Source: CAD feature listing. Evaluate the final solid. Frame: model axes, mm. Give positions to 0.01 mm unless a question says otherwise; leave off trailing zeros. Order: outer loops, then holes, each group sorted by start corner. A loop starts at its lowest first (then second) coordinate and runs counter-clockwise, first axis right, second up.
from build123d import *

# Parameters (mm, degrees)
BOSS_EXTRUDE1_DEPTH = 3.81
SKETCH2_R           = 3.175
CUT_EXTRUDE1_DEPTH  = 85.852


with BuildPart() as part:
    # Sketch1 → Boss-Extrude1 (new body)
    with BuildSketch(Plane(origin=(0, 0, 0), x_dir=(1, 0, 0), z_dir=(0, 1, 0))):
        with BuildLine():
            Line((-106.328404832, 71.61361972), (-235.457093287, 71.61361972))
            ThreePointArc((-235.457093287, 71.61361972), (-253.237093287, 53.83361972), (-235.457093287, 36.05361972))
            Line((-235.457093287, 36.05361972), (-215.137093287, 36.05361972))
            ThreePointArc((-215.137093287, 36.05361972), (-211.544990839, 34.565722168), (-210.057093287, 30.97361972))
            Line((-210.057093287, 30.97361972), (-210.057093287, -116.34638028))
            ThreePointArc((-210.057093287, -116.34638028), (-211.544990839, -119.938482729), (-215.137093287, -121.42638028))
            Line((-215.137093287, -121.42638028), (-235.457093287, -121.42638028))
            ThreePointArc((-235.457093287, -121.42638028), (-253.237093287, -139.20638028), (-235.457093287, -156.98638028))
            Line((-235.457093287, -156.98638028), (-106.328404832, -156.98638028))
            Line((-106.328404832, -156.98638028), (160.782906713, -156.98638028))
            Line((160.782906713, -156.98638028), (186.182906713, -156.98638028))
            ThreePointArc((186.182906713, -156.98638028), (203.962906713, -139.20638028), (186.182906713, -121.42638028))
            Line((186.182906713, -121.42638028), (165.862906713, -121.42638028))
            ThreePointArc((165.862906713, -121.42638028), (162.270804264, -119.938482729), (160.782906713, -116.34638028))
            Line((160.782906713, -116.34638028), (160.782906713, 30.97361972))
            ThreePointArc((160.782906713, 30.97361972), (162.270804264, 34.565722168), (165.862906713, 36.05361972))
            Line((165.862906713, 36.05361972), (186.182906713, 36.05361972))
            ThreePointArc((186.182906713, 36.05361972), (203.962906713, 53.83361972), (186.182906713, 71.61361972))
            Line((186.182906713, 71.61361972), (160.782906713, 71.61361972))
            Line((160.782906713, 71.61361972), (-106.328404832, 71.61361972))
        make_face()
    extrude(amount=BOSS_EXTRUDE1_DEPTH)

    # Sketch2 → Cut-Extrude1 (cut)
    with BuildSketch(Plane(origin=(0, 3.81, 0), x_dir=(1, 0, 0), z_dir=(0, 1, 0))):
        with Locations((-235.457093287, 53.83361972)):
            Circle(SKETCH2_R)
        with Locations((186.182906713, 53.83361972)):
            Circle(SKETCH2_R)
        with Locations((186.182906713, -139.20638028)):
            Circle(SKETCH2_R)
        with Locations((-235.457093287, -139.20638028)):
            Circle(SKETCH2_R)
    extrude(amount=-CUT_EXTRUDE1_DEPTH, mode=Mode.SUBTRACT)


solid = part.part
1) First-contact query: pin 1 Ø4 at (x, z) = (-235.46, 139.21) entering from +Y; pin 2 Ø5 at (x, z) = (-48, -15.5) entering from -Y. Flat tips, straight axial feed; report the tip coordinate or a pass-through.
Checks:
pin 1: passes through
pin 2: stops at y = 0
2) Section query C-C on z = 127. Output: boundary loops of the cut face in (x, y), and give its area (3 significant figures).
Checks:
outline: (-248.39, 0) - (199.11, 0) - (199.11, 3.81) - (-248.39, 3.81) - close
area: 1,700 mm2
3) Ray query, L1, parallel to X at y = 0.9, z = 142; L2, parallel to X at y = 2, z = -16; L3, parallel to X at y = 1.4, z = -47.5. Return the intervals inside material, ascending.
Checks:
L1: x = -253.02 to -236.97, -233.95 to 184.67, 187.69 to 203.74
L2: x = -210.06 to 160.78
L3: x = -252.07 to 202.8
4) Section query B-B on z = 1. Output: boundary loops of the cut face in (x, y), and give its area (3 significant figures).
Checks:
outline: (-210.06, 0) - (160.78, 0) - (160.78, 3.81) - (-210.06, 3.81) - close
area: 1,410 mm2
5) Section query A-A on y = 2.5. Output: boundary loops of the cut face in (x, z) (3 decimals), and give its area (3 significant figures).
Checks:
outline: (-235.457, -71.614) - (186.183, -71.614) arc R17.78 ccw to (186.183, -36.054) - (165.863, -36.054) arc R5.08 cw to (160.783, -30.974) - (160.783, 116.346) arc R5.08 cw to (165.863, 121.426) - (186.183, 121.426) arc R17.78 ccw to (186.183, 156.986) - (-235.457, 156.986) arc R17.78 ccw to (-235.457, 121.426) - (-215.137, 121.426) arc R5.08 cw to (-210.057, 116.346) - (-210.057, -30.974) arc R5.08 cw to (-215.137, -36.054) - (-235.457, -36.054) arc R17.78 ccw to start; hole circle Ø6.35 at (-235.457, -53.834); hole circle Ø6.35 at (-235.457, 139.206); hole circle Ø6.35 at (186.183, -53.834); hole circle Ø6.35 at (186.183, 139.206)
area: 90,300 mm2
6) Pull-direction query (Z, two-part tool) for faces 1 (the face through (203.96, 1.88, -53.44)), 2 (the face through (-28, 0, 41)); classes: +Z half, -Z half, draft (parallel to the pull), parting line (faces both ways), or undercut.
Checks:
face 1: undercut
face 2: draft
